Check sheet for the modelled part. Datum: model origin and axes. Units: mm. A direction names the side the tool comes from. Round coordinates to 2 decimals unless told otherwise and drop trailing zeros. Order: outer loops, then holes, each group sorted by start corner. A loop starts at its lowest first (then second) coordinate and runs counter-clockwise, first axis right, second up.
Autodesk Inventor part; units mm, degrees
ref_plane "YZ Plane" through (0, 0, 0) normal (1, 0, 0) x (0, 1, 0)
ref_plane "XZ Plane" through (0, 0, 0) normal (0, 1, 0) x (-1, 0, 0)
ref_plane "XY Plane" through (0, 0, 0) normal (0, 0, 1) x (1, 0, 0)
sketch "Sketch1" plane through (0, 0, 0) normal (0, 0, 1) x (1, 0, 0)
  line L0 (-9.525, -25.4) -> (9.525, -25.4)
  line L1 (9.525, -25.4) -> (9.525, 25.4)
  line L2 (9.525, 25.4) -> (-9.525, 25.4)
  line L3 (-9.525, 25.4) -> (-9.525, -25.4)
  line L4 (-9.525, -25.4) -> (9.525, 25.4) construction
  line L5 (9.525, -25.4) -> (-9.525, 25.4) construction
  line L6 (9.525, 25.4) -> (-9.525, 44.45)
  line L7 (-9.525, 44.45) -> (-9.525, 25.4)
  line L8 (-9.525, -25.4) -> (-9.525, -44.45)
  line L9 (-9.525, -44.45) -> (9.525, -25.4)
  point P0 (0, 0)
  dimension "d0" = 19.05
  dimension "d1" = 45
  dimension "d2" = 45
  dimension "d10" = 88.9
extrude "Extrusion1" add sketch "Sketch1" along normal mid plane 38.1
sketch "Sketch2" plane through (0, 0, 0) normal (0, 1, 0) x (-1, 0, 0)
  line L0 (6.35, 15.875) -> (-6.35, 15.875)
  line L1 (-6.35, 15.875) -> (-6.35, -15.875)
  line L2 (-6.35, -15.875) -> (6.35, -15.875)
  line L3 (6.35, -15.875) -> (6.35, 15.875)
  line L4 (6.35, 15.875) -> (-6.35, -15.875) construction
  line L5 (-6.35, 15.875) -> (6.35, -15.875) construction
  line L6 (-9.525, -19.05) -> (-9.525, 19.05)
  line L7 (-9.525, -19.05) -> (9.525, -19.05)
  point P0 (0, 0)
  dimension "d6" = 3.175
  dimension "d7" = 3.175
extrude "Extrusion2" cut sketch "Sketch2" along normal through all both and the other way through all
equation "\"d0\" = width"
equation "\"d10\" = length"
equation "\"d3\" = longSide"
equation "\"d8\" = longSide"
equation "\"width\" = 19.05"
equation "\"longSide\" = 38.1"
equation "\"length\" = 88.9"
properties part number "45dege0_75x1.50ForTopOfShooter" material "Aluminum 6061"
Item 1: Go/stop test with flat-tipped pins: P1, Ø1.5, axis at y = 33, z = -14, coming from the +X side; P2, Ø1, axis at x = -7.5, z = -4.5, coming from the -Y side (3 decimals); P3, Ø5, axis at x = -3, z = -11.5, coming from the +Y side. Record where each tip stops, or that it passes through.
Answer:
P1: stops at x = -6.35
P2: stops at y = -42.925
P3: passes through
Item 2: Scan lines: line 1 along X through (y, z) = (15.5, -8.5) (3 decimals); line 2 along Z through (x, y) = (5, 23.5) (3 decimals); line 3 along X through (y, z) = (-38.5, 1) (3 decimals). Record each from-to range of solid material in increasing order.
Answer:
line 1: x = -9.525 to -6.35, 6.35 to 9.525
line 2: z = -19.05 to -15.875, 15.875 to 19.05
line 3: x = -9.525 to -6.35
Item 3: Sectioned sample at A-A (z = 9). Record the cut outline in (x, y) (3 decimals), and give its area (3 significant figures).
Answer:
outline: (-9.525, -44.45) - (-6.35, -41.275) - (-6.35, 41.275) - (-9.525, 44.45) - close; (6.35, -28.575) - (9.525, -25.4) - (9.525, 25.4) - (6.35, 28.575) - close
area: 444 mm2
Item 4: Sectioned sample at C-C (x = 1.5). Record the cut outline in (y, z) (3 decimals), and give its area (3 significant figures).
Answer:
outline: (-33.425, -19.05) - (33.425, -19.05) - (33.425, -15.875) - (-33.425, -15.875) - close; (-33.425, 15.875) - (33.425, 15.875) - (33.425, 19.05) - (-33.425, 19.05) - close
area: 424 mm2
Item 5: Sectioned sample at D-D (x = -8). Record the cut outline in (y, z) (3 decimals), and give its area (3 significant figures).
Answer:
outline: (-42.925, -19.05) - (42.925, -19.05) - (42.925, 19.05) - (-42.925, 19.05) - close
area: 3,270 mm2
Item 6: Access from +Z, -Z, +X, -X, +Y, -Y to the whole of each face (thin tool, end or side, straight path). Record for faces 1 (the flat face through (-6.483, -41.408, -0.267)), 2 (the flat face through (6.35, 0, 0)).
Answer:
face 1: +Z, -Z, +X, -Y
face 2: +Y, -Y
Item 7: Release check for a two-part mould opening along Z. For faces 3 (the flat face through (-9.525, 1, 0)), 4 (the flat face through (-6.35, -1, 0)), 5 (the flat face through (0, 1, -19.05)), 6 (the flat face through (0, 1, 19.05)) record: released by +Z, released by -Z, zero draft, split by the parting line, or undercut.
Answer:
face 3: zero draft
face 4: undercut
face 5: released by -Z
face 6: released by +Z
Item 8: Sectioned sample at B-B (y = 10.5). Record the cut outline in (x, z) (3 decimals).
Answer:
outline: (-9.525, -19.05) - (9.525, -19.05) - (9.525, 19.05) - (-9.525, 19.05) - close; hole (-6.35, -15.875) - (6.35, -15.875) - (6.35, 15.875) - (-6.35, 15.875) - close
